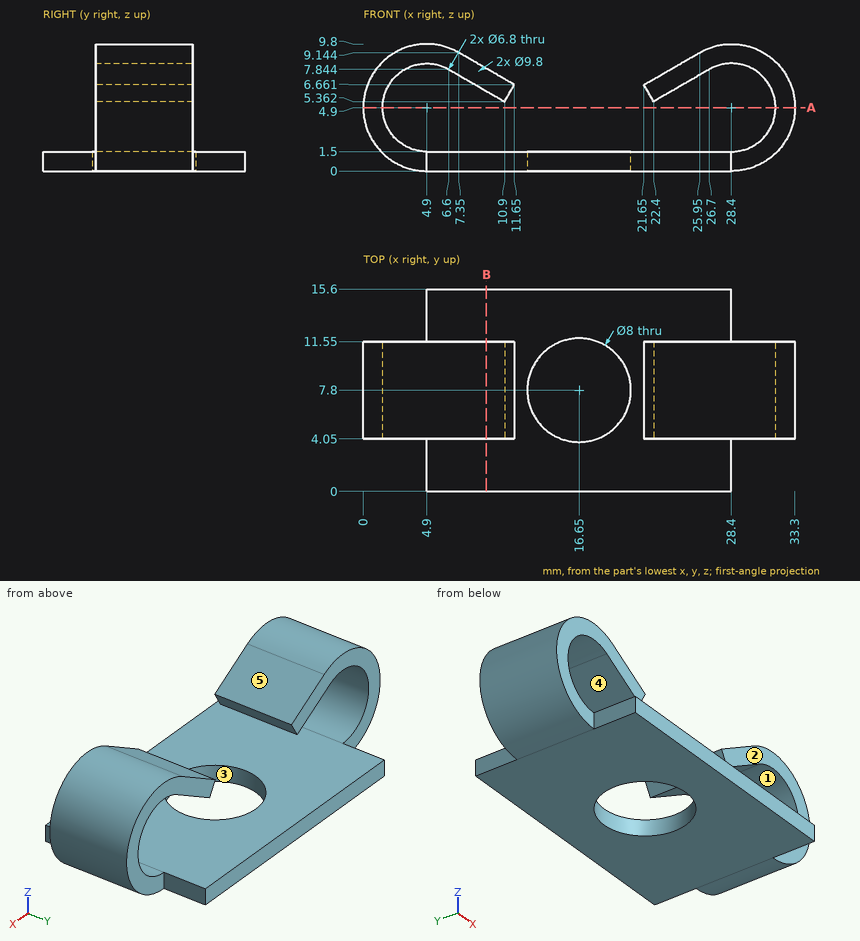
Geometry check sheet. Reference: drawing and pictorial views, mm from the part's lowest x, y, z. A direction names the side the tool comes from. Round coordinates to 2 decimals unless told otherwise and drop trailing zeros. Write each loop counter-clockwise with the first axis right and the second up, starting at its lowest first coordinate (ties: lowest second). Pieces come first, ordered by that corner, then holes. Notation, with made-up numbers: (69, 60) -> (101, 60) arc R14 cw to (101, 71) -> close; hole circle Ø6 at (57.5, 75.5). An arc over 180 degrees is marked (long way). Answer as CSV lines item,"result". Start each with the question number.
1) Material ranges on line 1 (X direction, y = 6.75, z = 4.9); line 2 (Y direction, x = 16.65, z = 0.65); line 3 (X direction, y = 9, z = 7) (1 decimal), recorded low to high. Write a range as from..to.
2) Go/stop test with flat-tipped pins: P1, Ø1, axis at x = 21.5, y = 7.5, coming from the -Z side; P2, Ø3, axis at y = 10.5, z = 3, coming from the +X side; P3, Ø5, axis at x = 4, z = 4, coming from the -Y side; P4, Ø1.5, axis at x = 10, z = 5.5, coming from the -Y side. Record where each tip stops, or that it passes through.
3) Section check A-A on z = 4.9. Enter the section's corners in (x, y).
4) Release check for a two-part mould opening along X. For the marked faces 1 and 2 record: pulls with the +X half, pulls with the -X half, needs draft (parallel to the pull), parting line crosses it, or undercut.
5) Tool access check on the marked faces 3, 4 and 5. Record the directions out of +Z, -Z, +X, -X, +Y, -Y that give a thin tool (end or side, any length) a straight path to the whole face; none if there is none.
6) Section check B-B on x = 9.5. Enter the section's corners in (y, z).
Found:
1,line 1,"x = 0..1.5, 31.8..33.3"
1,line 2,"y = 0..3.8, 11.8..15.6"
1,line 3,"x = 0.5..2.2, 8.1..11.1, 22.2..25.2, 31.1..32.8"
2,P1,"stops at z = 0"
2,P2,"stops at x = 33.28"
2,P3,"stops at y = 4.05"
2,P4,"stops at y = 4.05"
3,outline,"(0, 4.05) -> (1.5, 4.05) -> (1.5, 11.55) -> (0, 11.55) -> close; (31.8, 4.05) -> (33.3, 4.05) -> (33.3, 11.55) -> (31.8, 11.55) -> close"
4,face 1,"undercut"
4,face 2,"needs draft"
5,face 3,"+Z, -Z"
5,face 4,"+Y, -Y"
5,face 5,"+Z, +Y, -Y"
6,outline,"(0, 0) -> (15.6, 0) -> (15.6, 1.5) -> (0, 1.5) -> close; (4.05, 6.17) -> (11.55, 6.17) -> (11.55, 7.9) -> (4.05, 7.9) -> close"
